```python
from build123d import *

# Parameters (mm, degrees)
CHAMFER1_SIZE = 0.3


with BuildPart() as part:
    # Sketch1 → Revolve1 (revolve)
    with BuildSketch(Plane.XY, mode=Mode.PRIVATE) as revolve1_sk:
        Polygon((0, 6), (0, 10.5), (3, 10.5), (3, 8.5), (10, 8.5), (10, 6), align=None)
    revolve(revolve1_sk.sketch.rotate(Axis((0, 0, 0), (1, 0, 0)), 90), axis=Axis((0, 0, 0), (1, 0, 0)))

    # Chamfer1
    chamfer1_edges = [part.edges().sort_by_distance(p)[0] for p in [
        (10, 0, -6),
        (10, 0, -8.5),
        (3, 0, -10.5),
        (0, 0, -10.5),
        (0, 0, -6),
    ]]
    chamfer(chamfer1_edges, length=CHAMFER1_SIZE)


solid = part.part
```
Build history of the part. All positions in model axes, mm. A direction names the side the tool comes from. Give positions to 0.01 mm unless a question says otherwise; leave off trailing zeros. Loops run counter-clockwise (first coordinate to the right, second up) from the corner with the lowest first, then second, coordinate; pieces in that order, holes last.
Item 1: Which spindle directions (+Z, -Z, +X, -X, +Y, -Y) get a long thin tool onto all of the face, cutting with end or side? Do faces 4 (the face through (10, 6, 2.4)), 5 (the face through (6.397, -8.428, -1.107)). Say none if no direction does.
Answers follow:
face 4: +Z, -Z, +X, +Y, -Y
face 5: +X
Item 2: Slice it at D-D, the plane x = 1.75. List the corners of the cut face in (y, z), and give its area (3 significant figures).
Answers follow:
outline: circle Ø21 at (0, 0); hole circle Ø12 at (0, 0)
area: 233 mm2
Item 3: Flat gauge pins, fed straight in: pin 1 (5 mm diameter, centred on x = 7, y = 1, fed in from +Z); pin 2 (5 mm diameter, centred on x = 6.5, z = 3, fed in from +Y); pin 3 (1.5 mm diameter, centred on x = 9, y = -6, fed in from +Z); pin 4 (10 mm diameter, centred on y = 1.5, z = 4, fed in from +X). Where does each tip first touch, or does it go through?
Answers follow:
pin 1: stops at z = 8.5
pin 2: stops at y = 8.49
pin 3: stops at z = 6.68
pin 4: stops at x = 10
Item 4: Pull direction Y, two halves, no side cores. Call faces 1 (the face through (0, 0, -7)), 2 (the face through (1.5, -3.2, 10)), 3 (the face through (4.934, -1.802, 5.723)): released by +Y, released by -Y, zero draft, split by the parting line, or undercut.
Answers follow:
face 1: zero draft
face 2: split by the parting line
face 3: undercut
Item 5: Slice it at A-A, the plane y = 0. List the corners of the cut face in (x, z).
Answers follow:
outline: (0, -10.2) - (0.3, -10.5) - (2.7, -10.5) - (3, -10.2) - (3, -8.5) - (9.7, -8.5) - (10, -8.2) - (10, -6.3) - (9.7, -6) - (0.3, -6) - (0, -6.3) - close; (0, 6.3) - (0.3, 6) - (9.7, 6) - (10, 6.3) - (10, 8.2) - (9.7, 8.5) - (3, 8.5) - (3, 10.2) - (2.7, 10.5) - (0.3, 10.5) - (0, 10.2) - close
Item 6: Drill centre lines: line 1 (Y direction, x = 7.5, z = 0); line 2 (Y direction, x = 1.75, z = -0.5); line 3 (Z direction, x = 3.25, y = -0.5). Where is each one in solid material? Low to high.
Answers follow:
line 1: y = -8.5 to -6, 6 to 8.5
line 2: y = -10.49 to -5.98, 5.98 to 10.49
line 3: z = -8.49 to -5.98, 5.98 to 8.49
Item 7: Slice it at C-C, the plane x = 4.5. List the corners of the cut face in (y, z), and give its area (3 significant figures).
Answers follow:
outline: circle Ø17 at (0, 0); hole circle Ø12 at (0, 0)
area: 114 mm2
